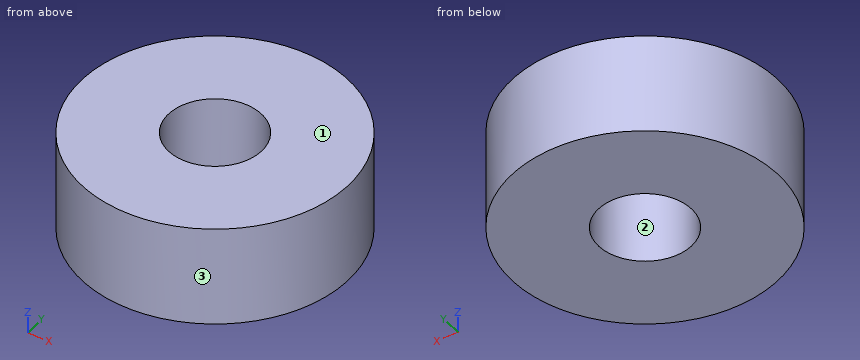
```python
from build123d import *

# Parameters (mm, degrees)
CYLINDER037_R     = 2.1
CYLINDER037_DEPTH = 33.5
CYLINDER036_R     = 6
CYLINDER036_DEPTH = 4.5


with BuildPart() as cylinder037:
    # Cylinder037 → Cylinder037 (new body)
    with BuildSketch(Plane.XY.offset(-4.6)):
        Circle(CYLINDER037_R)
    extrude(amount=CYLINDER037_DEPTH)


with BuildPart() as cut028:
    # Cylinder036 → Cylinder036 (new body)
    with BuildSketch(Plane.XY.offset(24)):
        Circle(CYLINDER036_R)
    extrude(amount=CYLINDER036_DEPTH)

    # Cut028: cut Cylinder037
    add(cylinder037.part, mode=Mode.SUBTRACT)


solid = cut028.part
```
Could you check a few things on this model? Use its own coordinates, in mm. Face numbers are marked on the shaded views. Round coordinates to 2 decimals unless told otherwise and drop trailing zeros. Loops run counter-clockwise (first coordinate to the right, second up) from the corner with the lowest first, then second, coordinate; pieces in that order, holes last. Notation, with made-up numbers: (81, -34.75) -> (120, -34.75) arc R22 ccw to (120, -9.75) -> close; hole circle Ø9 at (51, -12.5). An arc over 180 degrees is marked (long way). Put each result on its own line as item: value.
Q1. I want a section at D-D on x = -2.75. Write out the boundary of the cut face in (y, z).
Checks:
outline: (-5.33, 24) -> (5.33, 24) -> (5.33, 28.5) -> (-5.33, 28.5) -> close
Q2. Thinking about a two-plate mould opening in X: for the marked faces 1, 2 and 3, which applies, pulls with the +X half, pulls with the -X half, needs draft (parallel to the pull), parting line crosses it, or undercut?
Checks:
face 1: needs draft
face 2: undercut
face 3: parting line crosses it
Q3. Please list where these lines run through material, in increasing order: line 1 (Y direction, x = 0, z = 24.95); line 2 (X direction, y = 1.5, z = 26.05); line 3 (X direction, y = 1.75, z = 27.4). Write a range as from..to.
Checks:
line 1: -6..-2.1, 2.1..6
line 2: -5.81..-1.47, 1.47..5.81
line 3: -5.74..-1.16, 1.16..5.74
Q4. I want a section at C-C on z = 26.3. Write out the boundary of the cut face in (x, y), and give its area (3 significant figures).
Checks:
outline: circle Ø12 at (0, 0); hole circle Ø4.2 at (0, 0)
area: 99.2 mm2
Q5. I want a section at A-A on y = 0. Write out the boundary of the cut face in (x, z), and give its area (3 significant figures).
Checks:
outline: (-6, 24) -> (-2.1, 24) -> (-2.1, 28.5) -> (-6, 28.5) -> close; (2.1, 24) -> (6, 24) -> (6, 28.5) -> (2.1, 28.5) -> close
area: 35.1 mm2
Q6. For pin 1 Ø2 at (y, z) = (-1.5, 26.5) entering from -X; pin 2 Ø2 at (x, z) = (3.5, 27) entering from +Y; pin 3 Ø1.5 at (y, z) = (-4.5, 27) entering from -X; pin 4 Ø4 at (x, y) = (0, 0) entering from +Z, each with a flat end and sliding along its axis, tell me the tip position at first contact or that it passes through.
Checks:
pin 1: x = -5.98
pin 2: y = 5.45
pin 3: x = -4.68
pin 4: through
